Check sheet for the modelled part. Datum: model origin and axes. Units: mm. Round coordinates to 2 decimals unless told otherwise and drop trailing zeros. Order: outer loops, then holes, each group sorted by start corner. A loop starts at its lowest first (then second) coordinate and runs counter-clockwise, first axis right, second up. Notation, with made-up numbers: (14.25, 43) -> (54.25, 43) arc R23 cw to (54.25, 68) -> close; hole circle Ø10 at (40, -26.75). An arc over 180 degrees is marked (long way). Answer in a Markdown table with one row per item.
```python
from build123d import *

# Parameters (mm, degrees)
PIASTRAOUT_ESTRUSIONE_ESTRUSIONE1_START  = -1
PIASTRAOUT_ESTRUSIONE_ESTRUSIONE1_OUTL_R = 1.75
PIASTRAOUT_ESTRUSIONE_ESTRUSIONE1_DEPTH  = 1
SCHIZZO1_R                               = 6
TAGLIO_ESTRUSIONE1_DEPTH                 = 48.914602295
SCHIZZO2_R                               = 2.54
TAGLIO_ESTRUSIONE2_DEPTH                 = 48.914602295
SCHIZZO3_W                               = 29.718
SCHIZZO3_H                               = 11.938
TAGLIO_ESTRUSIONE3_DEPTH                 = 48.914602295


# Read off the part's stored shape, not the designer's step: <PiastraOUT>-<Estrusione-Estrusione1>
with BuildPart() as part:
    # <PiastraOUT>-<Estrusione-Estrusione1> outl → <PiastraOUT>-<Estrusione-Estrusione1> (new body)
    with BuildSketch(Plane.XY.offset(PIASTRAOUT_ESTRUSIONE_ESTRUSIONE1_START)):
        Polygon((-22.5, 3.708640208), (-22.5, -42.291359792), (22.5, -42.291359792), (22.5, 3.708640208), (12.5, 13.708640208), (-12.5, 13.708640208), align=None)
        with Locations((-10, -6.291359792)):
            Circle(PIASTRAOUT_ESTRUSIONE_ESTRUSIONE1_OUTL_R, mode=Mode.SUBTRACT)
        with Locations((-5, 8.708640208)):
            Circle(PIASTRAOUT_ESTRUSIONE_ESTRUSIONE1_OUTL_R, mode=Mode.SUBTRACT)
        with Locations((10, -6.291359792)):
            Circle(PIASTRAOUT_ESTRUSIONE_ESTRUSIONE1_OUTL_R, mode=Mode.SUBTRACT)
        with Locations((5, 8.708640208)):
            Circle(PIASTRAOUT_ESTRUSIONE_ESTRUSIONE1_OUTL_R, mode=Mode.SUBTRACT)
    extrude(amount=PIASTRAOUT_ESTRUSIONE_ESTRUSIONE1_DEPTH)

    # Schizzo1 → Taglio-Estrusione1 (cut, through all)
    with BuildSketch(Plane.XY):
        with Locations((5.74, -23.264939262)):
            Circle(SCHIZZO1_R)
    extrude(amount=-TAGLIO_ESTRUSIONE1_DEPTH, mode=Mode.SUBTRACT)

    # Schizzo2 → Taglio-Estrusione2 (cut, through all)
    with BuildSketch(Plane.XY):
        with Locations((-18.513603064, -23.499799375)):
            Circle(SCHIZZO2_R)
        with Locations((19.455356967, -23.132126406)):
            Circle(SCHIZZO2_R)
    extrude(amount=-TAGLIO_ESTRUSIONE2_DEPTH, mode=Mode.SUBTRACT)

    # Schizzo3 → Taglio-Estrusione3 (cut, through all)
    with BuildSketch(Plane.XY):
        with Locations((0.025, -23.264939262)):
            Rectangle(SCHIZZO3_W, SCHIZZO3_H)
    extrude(amount=-TAGLIO_ESTRUSIONE3_DEPTH, mode=Mode.SUBTRACT)


solid = part.part
```
(1) Section check D-D on z = -0.6. Record the boundary of the cut face in (x, y).
Solutions:
| item | result |
|---|---|
| outline | (-22.5, -42.29) -> (22.5, -42.29) -> (22.5, 3.71) -> (12.5, 13.71) -> (-12.5, 13.71) -> (-22.5, 3.71) -> close; hole circle Ø5.08 at (-18.51, -23.5); hole (-14.83, -29.23) -> (5.13, -29.23) arc R6 ccw to (6.35, -29.23) -> (14.88, -29.23) -> (14.88, -17.3) -> (6.35, -17.3) arc R6 ccw to (5.13, -17.3) -> (-14.83, -17.3) -> close; hole circle Ø3.5 at (-10, -6.29); hole circle Ø3.5 at (-5, 8.71); hole circle Ø3.5 at (5, 8.71); hole circle Ø3.5 at (10, -6.29); hole circle Ø5.08 at (19.46, -23.13) |
(2) Depth check by flat-ended pin: pin 1 Ø4.5 at (x, y) = (-18.51, -23.5) entering from +Z. Enter the tip coordinate at first touch or a pass-through.
Solutions:
| item | result |
|---|---|
| pin 1 | through |
(3) Section check C-C on x = 10. Record the boundary of the cut face in (y, z).
Solutions:
| item | result |
|---|---|
| outline | (-42.29, -1) -> (-29.23, -1) -> (-29.23, 0) -> (-42.29, 0) -> close; (-17.3, -1) -> (-8.04, -1) -> (-8.04, 0) -> (-17.3, 0) -> close; (-4.54, -1) -> (13.71, -1) -> (13.71, 0) -> (-4.54, 0) -> close |
(4) Section check A-A on y = -18.5. Record the boundary of the cut face in (x, z), plus the area to 3 significant figures.
Solutions:
| item | result |
|---|---|
| outline | (-22.5, -1) -> (-14.83, -1) -> (-14.83, 0) -> (-22.5, 0) -> close; (14.88, -1) -> (22.5, -1) -> (22.5, 0) -> (14.88, 0) -> close |
| area | 15.3 mm^2 |
(5) Section check B-B on x = 0. Record the boundary of the cut face in (y, z).
Solutions:
| item | result |
|---|---|
| outline | (-42.29, -1) -> (-29.23, -1) -> (-29.23, 0) -> (-42.29, 0) -> close; (-17.3, -1) -> (13.71, -1) -> (13.71, 0) -> (-17.3, 0) -> close |
(6) Scan lines: probe 1 along Y at (x, z) = (-10, -0.45); probe 2 along Y at (x, z) = (-5, -0.8); probe 3 along X at (y, z) = (-20, -0.1). Record each from-to range of solid material in increasing order. Write a range as from..to.
Solutions:
| item | result |
|---|---|
| probe 1 | -42.29..-29.23, -17.3..-8.04, -4.54..13.71 |
| probe 2 | -42.29..-29.23, -17.3..6.96, 10.46..13.71 |
| probe 3 | -22.5..-14.83, 14.88..22.5 |
(7) Draft check along X on faces 1 (the cylindrical face through (10.941, -4.816, -0.507)), 2 (the flat face through (-17.43, 8.78, -0.51)), 3 (the flat face through (0, -14, -1)). Enter one of: pulls with the +X half, pulls with the -X half, needs draft (parallel to the pull), parting line crosses it, or undercut.
Solutions:
| item | result |
|---|---|
| face 1 | undercut |
| face 2 | pulls with the -X half |
| face 3 | needs draft |
